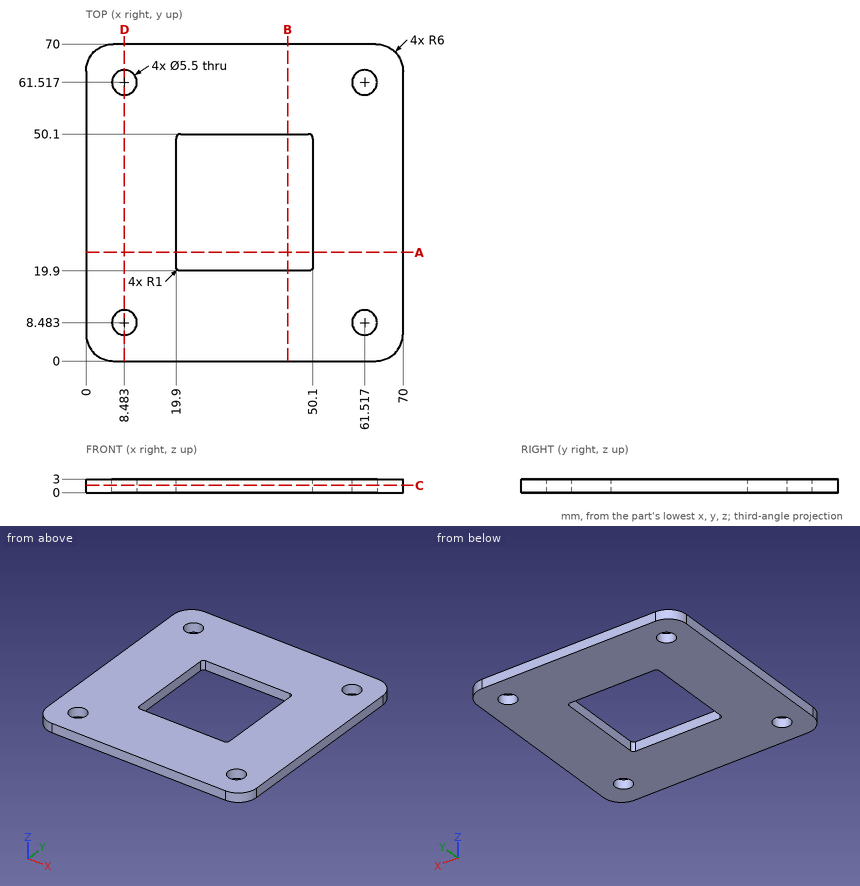
Part print with two shaded views. Sizes in mm from the minimum x, y, z corner. Coordinates: 2 decimals unless noted, no trailing zeros. Write each loop counter-clockwise with the first axis right and the second up, starting at its lowest first coordinate (ties: lowest second). Pieces come first, ordered by that corner, then holes. Notation, with made-up numbers: (71, 44.25) - (111, 44.25) arc R32 cw to (111, 80.25) - close; hole circle Ø6 at (72, 87). An arc over 180 degrees is marked (long way). Use a Markdown table: item, result. Add a question column.
Item 1: Drill centre lines: line 1 along X through (y, z) = (39, 1.35); line 2 along Y through (x, z) = (60.5, 0.25). Where is each one in solid material? Low to high.
Item 2: Band-saw the part on C-C, the plane z = 1.6. Write the cut outline in (x, y), and give its area (3 significant figures).
Item 3: Band-saw the part on D-D, the plane x = 8.5. Write the cut outline in (y, z), and give its area (3 significant figures).
Item 4: Band-saw the part on A-A, the plane y = 24. Write the cut outline in (x, z).
A:
| question | item | result |
|---|---|---|
| 1 | line 1 | x = 0 to 19.9, 50.1 to 70 |
| 1 | line 2 | y = 0 to 5.93, 11.04 to 58.96, 64.07 to 70 |
| 2 | outline | (0, 6) arc R6 ccw to (6, 0) - (64, 0) arc R6 ccw to (70, 6) - (70, 64) arc R6 ccw to (64, 70) - (6, 70) arc R6 ccw to (0, 64) - close; hole circle Ø5.5 at (8.48, 8.48); hole circle Ø5.5 at (8.48, 61.52); hole (19.9, 20.9) arc R1 ccw to (20.9, 19.9) - (49.1, 19.9) arc R1 ccw to (50.1, 20.9) - (50.1, 49.1) arc R1 ccw to (49.1, 50.1) - (20.9, 50.1) arc R1 ccw to (19.9, 49.1) - close; hole circle Ø5.5 at (61.52, 8.48); hole circle Ø5.5 at (61.52, 61.52) |
| 2 | area | 3,860 mm² |
| 3 | outline | (0, 0) - (5.73, 0) - (5.73, 3) - (0, 3) - close; (11.23, 0) - (58.77, 0) - (58.77, 3) - (11.23, 3) - close; (64.27, 0) - (70, 0) - (70, 3) - (64.27, 3) - close |
| 3 | area | 177 mm² |
| 4 | outline | (0, 0) - (19.9, 0) - (19.9, 3) - (0, 3) - close; (50.1, 0) - (70, 0) - (70, 3) - (50.1, 3) - close |
